```python
from build123d import *

# Parameters (mm, degrees)
SKETCH_2_W          = 40
SKETCH_2_H          = 40
SKETCH_2_W_2        = 20.3
SKETCH_2_H_2        = 20.3
EXTRUDE_1_DEPTH     = 94
CHAMFER_1_SIZE      = 2
CHAMFER_2_SIZE      = 2
SKETCH_5_R          = 1.25
CUT_EXTRUDE_2_DEPTH = 48
SKETCH_7_R          = 2.15
CUT_EXTRUDE_4_DEPTH = 79
CHAMFER_6_SIZE      = 1
SKETCH_8_W          = 65.895062616
SKETCH_8_H          = 54.143076927
CUT_EXTRUDE_5_DEPTH = 24
SKETCH_9_R          = 1.25
CUT_EXTRUDE_6_DEPTH = 49
CHAMFER_7_SIZE      = 1.5
CHAMFER_8_SIZE      = 2


with BuildPart() as part:
    # 草图2 → 凸台-拉伸1 (new body)
    with BuildSketch(Plane.XY):
        with Locations((20, 20)):
            Rectangle(SKETCH_2_W, SKETCH_2_H)
        with Locations((20, 20)):
            Rectangle(SKETCH_2_W_2, SKETCH_2_H_2, mode=Mode.SUBTRACT)
    extrude(amount=EXTRUDE_1_DEPTH)

    # 倒角1
    chamfer_1_edges = [part.edges().sort_by_distance(p)[0] for p in [
        (9.85, 20, 94),
        (20, 9.85, 94),
        (30.15, 20, 94),
        (20, 30.15, 94),
    ]]
    chamfer(chamfer_1_edges, length=CHAMFER_1_SIZE)

    # 倒角2
    chamfer_2_edges = [part.edges().sort_by_distance(p)[0] for p in [
        (0, 40, 47),
        (40, 40, 47),
        (40, 0, 47),
        (0, 0, 47),
    ]]
    chamfer(chamfer_2_edges, length=CHAMFER_2_SIZE)

    # 草图5 → 切除-拉伸2 (cut)
    with BuildSketch(Plane.XZ):
        with Locations(Location((20, 84, 0), (0, 0, 270))):
            Circle(SKETCH_5_R)
    extrude(amount=-CUT_EXTRUDE_2_DEPTH, mode=Mode.SUBTRACT)

    # 草图7 → 切除-拉伸4 (cut)
    with BuildSketch(Plane(origin=(40, 0, 0), x_dir=(0, 0, -1), z_dir=(1, 0, 0))):
        with Locations((-44, 20)):
            Circle(SKETCH_7_R)
    extrude(amount=-CUT_EXTRUDE_4_DEPTH, mode=Mode.SUBTRACT)

    # 倒角6
    chamfer_6_edges = [part.edges().sort_by_distance(p)[0] for p in [
        (0, 20, 46.15),
        (40, 20, 46.15),
    ]]
    chamfer(chamfer_6_edges, length=CHAMFER_6_SIZE)

    # 草图8 → 切除-拉伸5 (cut)
    with BuildSketch(Plane(origin=(0, 0, 0), x_dir=(-1, 0, 0), z_dir=(0, 0, -1))):
        with Locations((-18.489087128, 17.145946332)):
            Rectangle(SKETCH_8_W, SKETCH_8_H)
    extrude(amount=-CUT_EXTRUDE_5_DEPTH, mode=Mode.SUBTRACT)

    # 草图9 → 切除-拉伸6 (cut)
    with BuildSketch(Plane.ZY):
        with Locations((84, 20)):
            Circle(SKETCH_9_R)
    extrude(amount=-CUT_EXTRUDE_6_DEPTH, mode=Mode.SUBTRACT)

    # 倒角7
    chamfer_7_edges = [part.edges().sort_by_distance(p)[0] for p in [
        (30.15, 20, 82.75),
        (9.85, 20, 82.75),
        (20, 30.15, 85.25),
        (20, 9.85, 85.25),
    ]]
    chamfer(chamfer_7_edges, length=CHAMFER_7_SIZE)

    # 倒角8
    chamfer_8_edges = [part.edges().sort_by_distance(p)[0] for p in [
        (20, 9.85, 24),
        (9.85, 20, 24),
        (20, 30.15, 24),
        (30.15, 20, 24),
    ]]
    chamfer(chamfer_8_edges, length=CHAMFER_8_SIZE)


solid = part.part
```
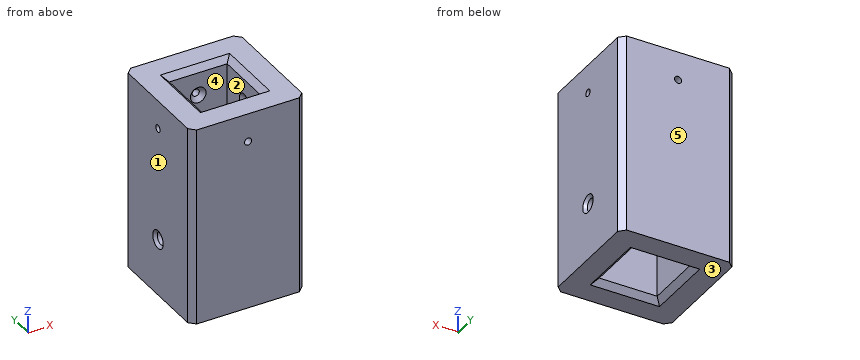
CAD build for the part. Positions are in the model's coordinates, mm. Face numbers are marked on the shaded views. A direction names the side the tool comes from. Round coordinates to 2 decimals unless told otherwise and drop trailing zeros. Order: outer loops, then holes, each group sorted by start corner. A loop starts at its lowest first (then second) coordinate and runs counter-clockwise, first axis right, second up.
Q1. Slice it at D-D (z = 29). Write the cut outline in (x, y).
Q2. Slice it at A-A (z = 44). Write the cut outline in (x, y), and give its area (3 significant figures).
Q3. Drop flat-ended pins along their axis: pin 1 (1.5 mm diameter, centred on x = 23.5, y = 30.5, fed in from -Z); pin 2 (5.5 mm diameter, centred on y = 20, z = 44, fed in from +X); pin 3 (3 mm diameter, centred on y = 20, z = 84, fed in from -X); pin 4 (5 mm diameter, centred on y = 20, z = 44, fed in from +X). Give the stop position or say it passes through.
Q4. Slice it at C-C (y = 12). Write the cut outline in (x, z).
Q5. Which spindle directions (+Z, -Z, +X, -X, +Y, -Y) get a long thin tool onto all of the face, cutting with end or side? Do the marked faces 1 and 2. Say none if no direction does.
Q6. Two-plate mould, pull along Y, no slides. Class the marked faces 3, 4 and 5: pulls with the +Y half, pulls with the -Y half, needs draft (parallel to the pull), parting line crosses it, or undercut.
Q7. Slice it at B-B (x = 20). Write the cut outline in (y, z), and give its area (3 significant figures).
Q8. Wall check: L1, parallel to X at y = 12, z = 69. Give the ranges that are in metal, low to high.
Results below:
1. outline: (0, 2) - (2, 0) - (38, 0) - (40, 2) - (40, 38) - (38, 40) - (2, 40) - (0, 38) - close; hole (9.85, 9.85) - (30.15, 9.85) - (30.15, 30.15) - (9.85, 30.15) - close
2. outline: (0, 2) - (2, 0) - (38, 0) - (40, 2) - (40, 16.85) - (39, 17.85) - (30.15, 17.85) - (30.15, 9.85) - (9.85, 9.85) - (9.85, 17.85) - (1, 17.85) - (0, 16.85) - close; (0, 23.15) - (1, 22.15) - (9.85, 22.15) - (9.85, 30.15) - (30.15, 30.15) - (30.15, 22.15) - (39, 22.15) - (40, 23.15) - (40, 38) - (38, 40) - (2, 40) - (0, 38) - close
2. area: 1,090 mm2
3. pin 1: stops at z = 24.9
3. pin 2: stops at x = 39.6
3. pin 3: stops at x = 0
3. pin 4: stops at x = 39.35
4. outline: (0, 24) - (7.85, 24) - (9.85, 26) - (9.85, 92) - (7.85, 94) - (0, 94) - close; (30.15, 26) - (32.15, 24) - (40, 24) - (40, 94) - (32.15, 94) - (30.15, 92) - close
5. face 1: +Z, -Z, -X, +Y, -Y
5. face 2: +Z, -Z
6. face 3: needs draft
6. face 4: undercut
6. face 5: pulls with the +Y half
7. outline: (0, 24) - (7.85, 24) - (9.85, 26) - (9.85, 81.25) - (8.35, 82.75) - (0, 82.75) - close; (0, 85.25) - (8.35, 85.25) - (9.85, 86.75) - (9.85, 92) - (7.85, 94) - (0, 94) - close; (30.15, 26) - (32.15, 24) - (40, 24) - (40, 82.75) - (31.65, 82.75) - (30.15, 81.25) - close; (30.15, 86.75) - (31.65, 85.25) - (40, 85.25) - (40, 94) - (32.15, 94) - (30.15, 92) - close
7. area: 1,320 mm2
8. L1: x = 0 to 9.85, 30.15 to 40
